```python
from build123d import *

# Parameters (mm, degrees)
F1_DEPTH = 6.35
F3_DEPTH = 50.8
F5_DEPTH = 76.2
F6_R     = 1.27
F7_DEPTH = 76.2


with BuildPart() as f1:
    # F0 (on Top) → F1 (new body)
    with BuildSketch(Plane.XY):
        with BuildLine():
            Line((43.18, 38.1), (-43.18, 38.1))
            ThreePointArc((-43.18, 38.1), (-48.5681536726, 35.8681536726), (-50.8, 30.48))
            Line((-50.8, 30.48), (-50.8, -30.48))
            ThreePointArc((-50.8, -30.48), (-48.5681536726, -35.8681536726), (-43.18, -38.1))
            Line((-43.18, -38.1), (43.18, -38.1))
            ThreePointArc((43.18, -38.1), (48.5681536726, -35.8681536726), (50.8, -30.48))
            Line((50.8, -30.48), (50.8, 30.48))
            ThreePointArc((50.8, 30.48), (48.5681536726, 35.8681536726), (43.18, 38.1))
        make_face()
    extrude(amount=F1_DEPTH)

    # F2 (on Top) → F3 (join)
    with BuildSketch(Plane.XY):
        with BuildLine():
            Line((-50.8, 30.48), (-50.8, -30.48))
            ThreePointArc((-50.8, -30.48), (-48.5681536726, -35.8681536726), (-43.18, -38.1))
            Line((-43.18, -38.1), (43.18, -38.1))
            ThreePointArc((43.18, -38.1), (48.5681536726, -35.8681536726), (50.8, -30.48))
            Line((50.8, -30.48), (50.8, 30.48))
            ThreePointArc((50.8, 30.48), (48.5681536726, 35.8681536726), (43.18, 38.1))
            Line((43.18, 38.1), (-43.18, 38.1))
            ThreePointArc((-43.18, 38.1), (-48.5681536726, 35.8681536726), (-50.8, 30.48))
        make_face()
        with BuildLine():
            Line((-46.99, -30.48), (-46.99, 30.48))
            ThreePointArc((-46.99, 30.48), (-45.5021024484, 34.0721024484), (-41.91, 35.56))
            Line((-41.91, 35.56), (41.91, 35.56))
            ThreePointArc((41.91, 35.56), (45.5021024484, 34.0721024484), (46.99, 30.48))
            Line((46.99, 30.48), (46.99, -30.48))
            ThreePointArc((46.99, -30.48), (45.5021024484, -34.0721024484), (41.91, -35.56))
            Line((41.91, -35.56), (-41.91, -35.56))
            ThreePointArc((-41.91, -35.56), (-45.5021024484, -34.0721024484), (-46.99, -30.48))
        make_face(mode=Mode.SUBTRACT)
    extrude(amount=F3_DEPTH)

    # F4 (on face) → F5 (join)
    with BuildSketch(Plane.XY.offset(6.35)):
        with BuildLine():
            Line((41.91, 35.56), (-41.91, 35.56))
            ThreePointArc((-41.91, 35.56), (-45.5021024484, 34.0721024484), (-46.99, 30.48))
            Line((-46.99, 30.48), (-46.99, -30.48))
            ThreePointArc((-46.99, -30.48), (-45.5021024484, -34.0721024484), (-41.91, -35.56))
            Line((-41.91, -35.56), (41.91, -35.56))
            ThreePointArc((41.91, -35.56), (45.5021024484, -34.0721024484), (46.99, -30.48))
            Line((46.99, -30.48), (46.99, 30.48))
            ThreePointArc((46.99, 30.48), (45.5021024484, 34.0721024484), (41.91, 35.56))
        make_face()
    extrude(amount=F5_DEPTH)

    # F6 (on face) → F7 (cut)
    with BuildSketch(Plane.XY.offset(82.55)):
        with BuildLine():
            Line((46.99, -30.48), (46.99, 30.48))
            ThreePointArc((46.99, 30.48), (45.5021024484, 34.0721024484), (41.91, 35.56))
            Line((41.91, 35.56), (-41.91, 35.56))
            ThreePointArc((-41.91, 35.56), (-45.5021024484, 34.0721024484), (-46.99, 30.48))
            Line((-46.99, 30.48), (-46.99, -30.48))
            ThreePointArc((-46.99, -30.48), (-45.5021024484, -34.0721024484), (-41.91, -35.56))
            Line((-41.91, -35.56), (41.91, -35.56))
            ThreePointArc((41.91, -35.56), (45.5021024484, -34.0721024484), (46.99, -30.48))
        make_face()
        with Locations((-40.6371347628, -29.3689621186)):
            Circle(F6_R, mode=Mode.SUBTRACT)
        with Locations((-31.6196572232, -29.2684558051)):
            Circle(F6_R, mode=Mode.SUBTRACT)
        with Locations((-40.5106123023, -21.0874684322)):
            Circle(F6_R, mode=Mode.SUBTRACT)
        with Locations((-31.4931347628, -20.9869621186)):
            Circle(F6_R, mode=Mode.SUBTRACT)
        with Locations((-22.6021796837, -29.1679494915)):
            Circle(F6_R, mode=Mode.SUBTRACT)
        with Locations((-13.5847021441, -29.0674431779)):
            Circle(F6_R, mode=Mode.SUBTRACT)
        with Locations((-4.5672246046, -28.9669368644)):
            Circle(F6_R, mode=Mode.SUBTRACT)
        with Locations((-22.4756572232, -20.8864558051)):
            Circle(F6_R, mode=Mode.SUBTRACT)
        with Locations((-13.4581796837, -20.7859494915)):
            Circle(F6_R, mode=Mode.SUBTRACT)
        with Locations((-4.4407021441, -20.6854431779)):
            Circle(F6_R, mode=Mode.SUBTRACT)
        with Locations((-40.3840898418, -12.8059747458)):
            Circle(F6_R, mode=Mode.SUBTRACT)
        with Locations((-31.3666123023, -12.7054684322)):
            Circle(F6_R, mode=Mode.SUBTRACT)
        with Locations((-40.2575673814, -4.5244810593)):
            Circle(F6_R, mode=Mode.SUBTRACT)
        with Locations((-31.2400898418, -4.4239747458)):
            Circle(F6_R, mode=Mode.SUBTRACT)
        with Locations((-22.3491347628, -12.6049621186)):
            Circle(F6_R, mode=Mode.SUBTRACT)
        with Locations((-13.3316572232, -12.5044558051)):
            Circle(F6_R, mode=Mode.SUBTRACT)
        with Locations((-4.3141796837, -12.4039494915)):
            Circle(F6_R, mode=Mode.SUBTRACT)
        with Locations((-22.2226123023, -4.3234684322)):
            Circle(F6_R, mode=Mode.SUBTRACT)
        with Locations((-13.2051347628, -4.2229621186)):
            Circle(F6_R, mode=Mode.SUBTRACT)
        with Locations((-4.1876572232, -4.1224558051)):
            Circle(F6_R, mode=Mode.SUBTRACT)
        with Locations((4.4502529349, -28.8664305508)):
            Circle(F6_R, mode=Mode.SUBTRACT)
        with Locations((13.4677304745, -28.7659242373)):
            Circle(F6_R, mode=Mode.SUBTRACT)
        with Locations((22.485208014, -28.6654179237)):
            Circle(F6_R, mode=Mode.SUBTRACT)
        with Locations((4.5767753954, -20.5849368644)):
            Circle(F6_R, mode=Mode.SUBTRACT)
        with Locations((13.5942529349, -20.4844305508)):
            Circle(F6_R, mode=Mode.SUBTRACT)
        with Locations((22.6117304745, -20.3839242373)):
            Circle(F6_R, mode=Mode.SUBTRACT)
        with Locations((31.5026855536, -28.5649116101)):
            Circle(F6_R, mode=Mode.SUBTRACT)
        with Locations((40.5201630931, -28.4644052966)):
            Circle(F6_R, mode=Mode.SUBTRACT)
        with Locations((31.629208014, -20.2834179237)):
            Circle(F6_R, mode=Mode.SUBTRACT)
        with Locations((40.6466855536, -20.1829116101)):
            Circle(F6_R, mode=Mode.SUBTRACT)
        with Locations((4.7032978559, -12.3034431779)):
            Circle(F6_R, mode=Mode.SUBTRACT)
        with Locations((13.7207753954, -12.2029368644)):
            Circle(F6_R, mode=Mode.SUBTRACT)
        with Locations((22.7382529349, -12.1024305508)):
            Circle(F6_R, mode=Mode.SUBTRACT)
        with Locations((4.8298203163, -4.0219494915)):
            Circle(F6_R, mode=Mode.SUBTRACT)
        with Locations((13.8472978559, -3.9214431779)):
            Circle(F6_R, mode=Mode.SUBTRACT)
        with Locations((22.8647753954, -3.8209368644)):
            Circle(F6_R, mode=Mode.SUBTRACT)
        with Locations((31.7557304745, -12.0019242373)):
            Circle(F6_R, mode=Mode.SUBTRACT)
        with Locations((40.773208014, -11.9014179237)):
            Circle(F6_R, mode=Mode.SUBTRACT)
        with Locations((31.8822529349, -3.7204305508)):
            Circle(F6_R, mode=Mode.SUBTRACT)
        with Locations((40.8997304745, -3.6199242373)):
            Circle(F6_R, mode=Mode.SUBTRACT)
        with Locations((-40.1310449209, 3.7570126271)):
            Circle(F6_R, mode=Mode.SUBTRACT)
        with Locations((-31.1135673814, 3.8575189407)):
            Circle(F6_R, mode=Mode.SUBTRACT)
        with Locations((-40.0045224605, 12.0385063136)):
            Circle(F6_R, mode=Mode.SUBTRACT)
        with Locations((-30.9870449209, 12.1390126271)):
            Circle(F6_R, mode=Mode.SUBTRACT)
        with Locations((-22.0960898418, 3.9580252542)):
            Circle(F6_R, mode=Mode.SUBTRACT)
        with Locations((-13.0786123023, 4.0585315678)):
            Circle(F6_R, mode=Mode.SUBTRACT)
        with Locations((-4.0611347628, 4.1590378814)):
            Circle(F6_R, mode=Mode.SUBTRACT)
        with Locations((-21.9695673814, 12.2395189407)):
            Circle(F6_R, mode=Mode.SUBTRACT)
        with Locations((-12.9520898418, 12.3400252542)):
            Circle(F6_R, mode=Mode.SUBTRACT)
        with Locations((-3.9346123023, 12.4405315678)):
            Circle(F6_R, mode=Mode.SUBTRACT)
        with Locations((-39.878, 20.32)):
            Circle(F6_R, mode=Mode.SUBTRACT)
        with Locations((-30.8605224605, 20.4205063136)):
            Circle(F6_R, mode=Mode.SUBTRACT)
        with Locations((-39.7514775395, 28.6014936864)):
            Circle(F6_R, mode=Mode.SUBTRACT)
        with Locations((-30.734, 28.702)):
            Circle(F6_R, mode=Mode.SUBTRACT)
        with Locations((-21.8430449209, 20.5210126271)):
            Circle(F6_R, mode=Mode.SUBTRACT)
        with Locations((-12.8255673814, 20.6215189407)):
            Circle(F6_R, mode=Mode.SUBTRACT)
        with Locations((-3.8080898418, 20.7220252542)):
            Circle(F6_R, mode=Mode.SUBTRACT)
        with Locations((-21.7165224605, 28.8025063136)):
            Circle(F6_R, mode=Mode.SUBTRACT)
        with Locations((-12.6990449209, 28.9030126271)):
            Circle(F6_R, mode=Mode.SUBTRACT)
        with Locations((-3.6815673814, 29.0035189407)):
            Circle(F6_R, mode=Mode.SUBTRACT)
        with Locations((4.9563427768, 4.2595441949)):
            Circle(F6_R, mode=Mode.SUBTRACT)
        with Locations((13.9738203163, 4.3600505085)):
            Circle(F6_R, mode=Mode.SUBTRACT)
        with Locations((22.9912978559, 4.4605568221)):
            Circle(F6_R, mode=Mode.SUBTRACT)
        with Locations((5.0828652372, 12.5410378814)):
            Circle(F6_R, mode=Mode.SUBTRACT)
        with Locations((14.1003427768, 12.6415441949)):
            Circle(F6_R, mode=Mode.SUBTRACT)
        with Locations((23.1178203163, 12.7420505085)):
            Circle(F6_R, mode=Mode.SUBTRACT)
        with Locations((32.0087753954, 4.5610631356)):
            Circle(F6_R, mode=Mode.SUBTRACT)
        with Locations((41.0262529349, 4.6615694492)):
            Circle(F6_R, mode=Mode.SUBTRACT)
        with Locations((32.1352978559, 12.8425568221)):
            Circle(F6_R, mode=Mode.SUBTRACT)
        with Locations((41.1527753954, 12.9430631356)):
            Circle(F6_R, mode=Mode.SUBTRACT)
        with Locations((5.2093876977, 20.8225315678)):
            Circle(F6_R, mode=Mode.SUBTRACT)
        with Locations((14.2268652372, 20.9230378814)):
            Circle(F6_R, mode=Mode.SUBTRACT)
        with Locations((23.2443427768, 21.0235441949)):
            Circle(F6_R, mode=Mode.SUBTRACT)
        with Locations((5.3359101582, 29.1040252542)):
            Circle(F6_R, mode=Mode.SUBTRACT)
        with Locations((14.3533876977, 29.2045315678)):
            Circle(F6_R, mode=Mode.SUBTRACT)
        with Locations((23.3708652372, 29.3050378814)):
            Circle(F6_R, mode=Mode.SUBTRACT)
        with Locations((32.2618203163, 21.1240505085)):
            Circle(F6_R, mode=Mode.SUBTRACT)
        with Locations((41.2792978559, 21.2245568221)):
            Circle(F6_R, mode=Mode.SUBTRACT)
        with Locations((32.3883427768, 29.4055441949)):
            Circle(F6_R, mode=Mode.SUBTRACT)
        with Locations((41.4058203163, 29.5060505085)):
            Circle(F6_R, mode=Mode.SUBTRACT)
    extrude(amount=-F7_DEPTH, mode=Mode.SUBTRACT)


solid = f1.part
```
Here's how the part is built. I have some questions about the finished solid (model axes, mm). A direction names the side the tool comes from. Round coordinates to 2 decimals unless told otherwise and drop trailing zeros. Order: outer loops, then holes, each group sorted by start corner. A loop starts at its lowest first (then second) coordinate and runs counter-clockwise, first axis right, second up. Notation, with made-up numbers: (18, 34) -> (36, 34) arc R28 ccw to (36, 68) -> close; hole circle Ø11 at (89, 25). An arc over 180 degrees is marked (long way). Use a Markdown table: item, result. Add a question column.
(1) Suppose I cut it at C-C, the plane z = 20.5. Count the separate pieces of the cut face and the enclosed holes in it, and give its area (3 significant figures).
(2) Suppose I cut it at B-B, the plane y = -16. Please give me the cut outline in (x, z), and give its area (3 significant figures).
(3) For faces 4 (the face through (15.036, 30.275, 44.983)), 5 (the face through (41, 5, 82.55)), which set-ups out of +Z, -Z, +X, -X, +Y, -Y let a thin tool reach every point of the face, with its end or its side?
(4) For pin 1 Ø1 at (x, y) = (36, 6) entering from +Z; pin 2 Ø8 at (y, z) = (-15, 66.5) entering from -X, each with a flat end and sliding along its axis, tell me the tip position at first contact or that it passes through.
(5) If we mould it in two halves opening along X, with no side actions, what happens to faces 1 (the face through (-50.8, 0, 25)), 2 (the face through (-40.81, 21.18, 44.98)), 3 (the face through (-22, -4, 82.55))? For each: released by +X, released by -X, zero draft, split by the parting line, or undercut.
(6) Suppose I cut it at A-A, the plane x = -9.5. Please give me the cut outline in (y, z).
(7) I need wall thicknesses on line 1 along X through (y, z) = (-7, 46.5); line 2 along Y through (x, z) = (25, 33.5); line 3 along Z through (x, y) = (15.5, -14). Which ranges of each line are inside material? Lowest first, please.
Verdict:
| question | item | result |
|---|---|---|
| 1 | separate pieces | 81 |
| 1 | enclosed holes | 1 |
| 1 | area | 1,440 mm2 |
| 2 | outline | (-50.8, 0) -> (50.8, 0) -> (50.8, 50.8) -> (46.99, 50.8) -> (46.99, 6.35) -> (-46.99, 6.35) -> (-46.99, 50.8) -> (-50.8, 50.8) -> close |
| 2 | area | 984 mm2 |
| 3 | face 4 | +Z |
| 3 | face 5 | +Z, +X, -X, +Y, -Y |
| 4 | pin 1 | z = 6.35 |
| 4 | pin 2 | x = -41.65 |
| 5 | face 1 | released by -X |
| 5 | face 2 | undercut |
| 5 | face 3 | zero draft |
| 6 | outline | (-38.1, 0) -> (38.1, 0) -> (38.1, 50.8) -> (35.56, 50.8) -> (35.56, 6.35) -> (-35.56, 6.35) -> (-35.56, 50.8) -> (-38.1, 50.8) -> close |
| 7 | line 1 | -50.8 to -46.99, 46.99 to 50.8 |
| 7 | line 2 | -38.1 to -35.56, 35.56 to 38.1 |
| 7 | line 3 | 0 to 6.35 |
